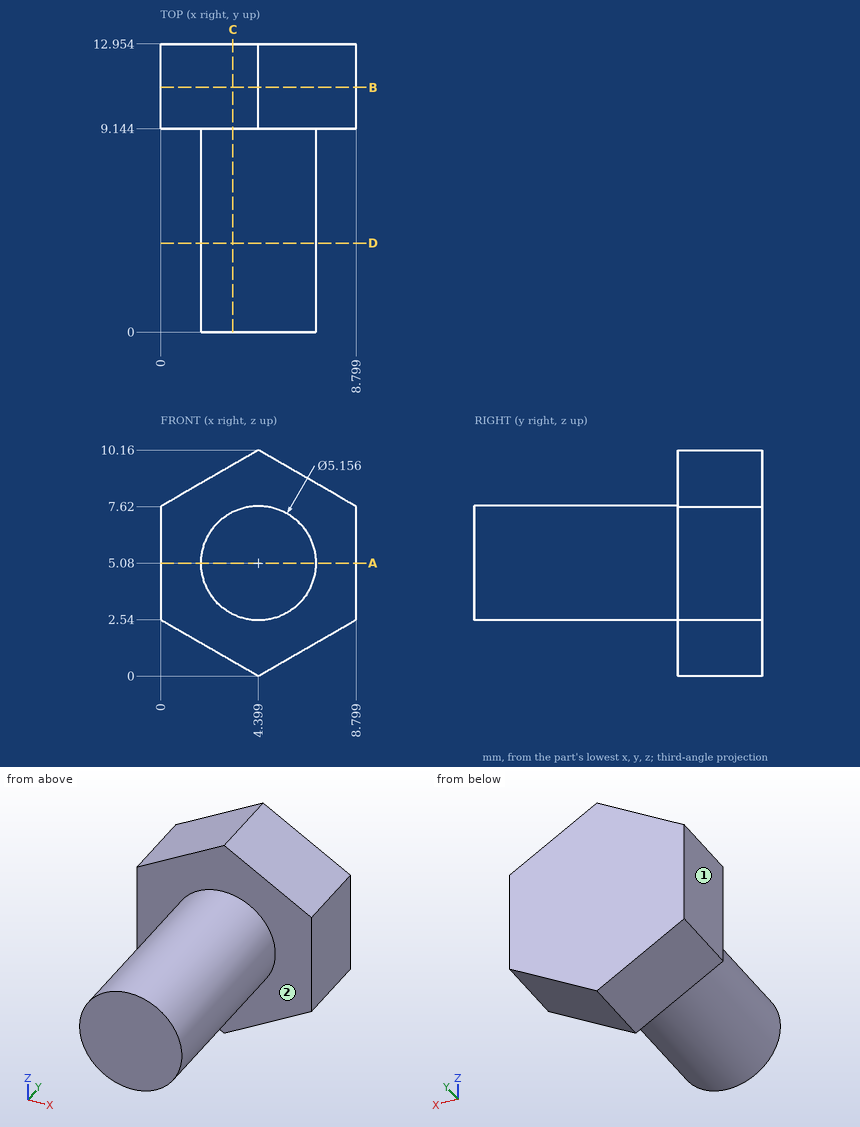
The figure shows three views and two pictorial views of one solid part (mm, origin at its lowest corner). Answer the questions. A direction names the side the tool comes from. Give positions to 0.01 mm unless a question says otherwise; leave off trailing zeros. Write each loop counter-clockwise with the first axis right and the second up, starting at its lowest first coordinate (ties: lowest second). Pieces come first, ordered by that corner, then holes.
Q1. Given pin 1 (2 mm diameter, centred on y = 3.5, z = 4.5, fed in from -X); pin 2 (4 mm diameter, centred on x = 2.5, y = 10.5, fed in from -Z), each flat-ended and moving along its own axis, determine where each tip first touches the part or whether it passes through.
Answer:
pin 1: stops at x = 1.82
pin 2: stops at z = 0
Q2. The part is cut by section B-B on y = 11. Give the vertices of the cut face in (x, z).
Answer:
outline: (0, 2.54) - (4.4, 0) - (8.8, 2.54) - (8.8, 7.62) - (4.4, 10.16) - (0, 7.62) - close
Q3. The part is cut by section A-A on z = 5.08. Give the vertices of the cut face in (x, y).
Answer:
outline: (0, 9.14) - (1.82, 9.14) - (1.82, 0) - (6.98, 0) - (6.98, 9.14) - (8.8, 9.14) - (8.8, 12.95) - (0, 12.95) - close
Q4. Straight lines are drawn through the part: L1, parallel to Y at x = 1.5, z = 2.75; L2, parallel to X at y = 5.75, z = 5; L3, parallel to X at y = 4, z = 3 (1 decimal). For each, find the intervals that lie inside material, in ascending order.
Answer:
L1: y = 9.14 to 12.95
L2: x = 1.82 to 6.98
L3: x = 2.9 to 5.9
Q5. A tool of negligible diameter and unlimited length cuts with its end or side. For the marked faces 1 and 2, from which of +Z, -Z, +X, -X, +Y, -Y can it reach the whole face along a straight path? Write none if from no direction.
Answer:
face 1: +Z, -Z, -X, +Y, -Y
face 2: -Y
Q6. The part is cut by section C-C on x = 3.25. Give the vertices of the cut face in (y, z).
Answer:
outline: (0, 2.77) - (9.14, 2.77) - (9.14, 0.66) - (12.95, 0.66) - (12.95, 9.5) - (9.14, 9.5) - (9.14, 7.39) - (0, 7.39) - close
Q7. The part is cut by section D-D on y = 4. Give the vertices of the cut face in (x, z), and give its area (3 significant figures).
Answer:
outline: circle Ø5.16 at (4.4, 5.08)
area: 20.9 mm2
